```python
from build123d import *

# Parameters (mm, degrees)
SKETCH2_W           = 59.055
SKETCH2_H           = 25.4
BOSS_EXTRUDE1_DEPTH = 2
BOSS_EXTRUDE2_START = 2
BOSS_EXTRUDE2_DEPTH = 9.525
SKETCH3_W           = 38.1
SKETCH3_H           = 25.4
BOSS_EXTRUDE3_DEPTH = 2
BOSS_EXTRUDE4_START = 2
SKETCH4_W           = 3.175
SKETCH4_H           = 25.4
BOSS_EXTRUDE4_DEPTH = 6.35
SKETCH5_R           = 1.5875
CUT_EXTRUDE1_DEPTH  = 3.175
SKETCH6_W           = 35.56
SKETCH6_H           = 71.12
SKETCH6_R           = 1.5875
BOSS_EXTRUDE5_DEPTH = 2
FILLET1_R           = 2.54
SKETCH10_R          = 13.129221829
CUT_EXTRUDE2_DEPTH  = 2


with BuildPart() as part:
    # Sketch2 → Boss-Extrude1 (new body)
    with BuildSketch(Plane(origin=(0, 0, 0), x_dir=(1, 0, 0), z_dir=(0, 1, 0))):
        with Locations((26.9875, 154.94)):
            Rectangle(SKETCH2_W, SKETCH2_H)
    extrude(amount=BOSS_EXTRUDE1_DEPTH)

    # Sketch1 → Boss-Extrude2 (add)
    with BuildSketch(Plane(origin=(0, 0, 0), x_dir=(1, 0, 0), z_dir=(0, 1, 0)).offset(BOSS_EXTRUDE2_START)):
        Polygon((-2.54, 167.64), (-2.54, 158.115), (0, 158.115), (0, 165.1), (53.975, 165.1), (53.975, 158.115), (56.515, 158.115), (56.515, 167.64), align=None)
    extrude(amount=BOSS_EXTRUDE2_DEPTH)

    # Sketch3 → Boss-Extrude3 (add)
    with BuildSketch(Plane(origin=(0, 0, 0), x_dir=(1, 0, 0), z_dir=(0, 1, 0))):
        with Locations((75.565, 154.94)):
            Rectangle(SKETCH3_W, SKETCH3_H)
    extrude(amount=BOSS_EXTRUDE3_DEPTH)

    # Sketch4 → Boss-Extrude4 (add)
    with BuildSketch(Plane(origin=(0, 0, 0), x_dir=(1, 0, 0), z_dir=(0, 1, 0)).offset(BOSS_EXTRUDE4_START)):
        with Locations((93.0275, 154.94)):
            Rectangle(SKETCH4_W, SKETCH4_H)
    extrude(amount=BOSS_EXTRUDE4_DEPTH)

    # Sketch5 → Cut-Extrude1 (cut)
    with BuildSketch(Plane(origin=(94.615, 0, 0), x_dir=(0, 0, -1), z_dir=(1, 0, 0))):
        with Locations((145.94, 4.895971622)):
            Circle(SKETCH5_R)
        with Locations(Location((163.94, 4.895971622, 0), (0, 0, 180))):
            Circle(SKETCH5_R)
    extrude(amount=-CUT_EXTRUDE1_DEPTH, mode=Mode.SUBTRACT)

    # Mirror1: part across plane


with BuildPart() as part_1:
    add(part.part)
    add(part.part.mirror(Plane(origin=(26.9875, 0, 0), x_dir=(0, 0, 1), z_dir=(1, 0, 0))))

    # Sketch6 → Boss-Extrude5 (add)
    with BuildSketch(Plane(origin=(0, 0, 0), x_dir=(1, 0, 0), z_dir=(0, 1, 0))):
        with Locations((26.9875, 203.2)):
            Rectangle(SKETCH6_W, SKETCH6_H)
        with Locations(Location((11.09051688, 236.783908574, 0), (0, 0, 270))):
            Circle(SKETCH6_R, mode=Mode.SUBTRACT)
        with Locations(Location((11.09051688, 205.176091426, 0), (0, 0, 90))):
            Circle(SKETCH6_R, mode=Mode.SUBTRACT)
        with Locations(Location((42.88448312, 205.176091426, 0), (0, 0, 270))):
            Circle(SKETCH6_R, mode=Mode.SUBTRACT)
        with Locations(Location((42.88448312, 236.783908574, 0), (0, 0, 90))):
            Circle(SKETCH6_R, mode=Mode.SUBTRACT)
    extrude(amount=BOSS_EXTRUDE5_DEPTH)

    # Fillet1
    fillet1_edges = [part_1.edges().sort_by_distance(p)[0] for p in [
        (26.9875, 2, -167.64),
    ]]
    fillet(fillet1_edges, radius=FILLET1_R)

    # Sketch10 → Cut-Extrude2 (cut)
    with BuildSketch(Plane(origin=(0, 2, 0), x_dir=(1, 0, 0), z_dir=(0, 1, 0))):
        with Locations(Location((26.9875, 224.917, 0), (0, 0, 270))):
            Circle(SKETCH10_R)
    extrude(amount=-CUT_EXTRUDE2_DEPTH, mode=Mode.SUBTRACT)


solid = part_1.part
```
Could you check a few things on this model? Use its own coordinates, in mm. A direction names the side the tool comes from. Round coordinates to 2 decimals unless told otherwise and drop trailing zeros. Write each loop counter-clockwise with the first axis right and the second up, starting at its lowest first coordinate (ties: lowest second). Pieces come first, ordered by that corner, then holes. Notation, with made-up numbers: M -9.75,5 L 7.25,5 A32 cw 7.25,41 Z; hole C 17.25,77 d8. An arc over 180 degrees is marked long. Answer in a Markdown table with one row per item. Add a question column.
Q1. Imagine slicing it at C-C (z = -188.5). Please give me the cut outline in (x, y), then the cut area to 3 significant figures.
Q2. Will these pins go through, and if not, where does the flat tip stop? pin 1 Ø1 at (x, z) = (-38.5, -151.5) entering from +Y; pin 2 Ø3.5 at (y, z) = (4.9, -163.94) entering from -X; pin 3 Ø3 at (x, y) = (36.5, 8) entering from +Z; pin 4 Ø3 at (y, z) = (4.9, -163.94) entering from -X.
Q3. Imagine slicing it at A-A (z = -145.94). Please give me the cut outline in (x, y) (3 decimals), then the cut area to 3 significant figures.
Q4. If we mould it in two halves opening along X, with no side actions, what happens to faces 4 (the cylindrical face through (11.57, 0.99, -235.27)), 5 (the flat face through (44.768, 1, -203)), 6 (the cylindrical face through (93.05, 4.966, -144.354)), 7 (the flat face through (56.515, 7, -163))? For each: +X half, -X half, draft (parallel to the pull), parting line (faces both ways), or undercut.
Q5. Imagine slicing it at B-B (z = -232). Please give me the cut outline in (x, y).
Q6. Imagine slicing it at D-D (x = -21). Please give me the cut outline in (y, z).
Q7. If I drill on line 1 (X direction, y = 7.75, z = -163) (3 decimals); line 2 (Y direction, x = 38, z = -207.5); line 3 (Z direction, x = 6, y = 5.75), over which ranges is the centre line in solid material (lowest first)? Write a range as from..to.
Q8. On a 3-axis mill with a long thin cutter (end or side, diameter ignored), from which of +Z, -Z, +X, -X, +Y, -Y can I reach the whole of each face in a straight line? I mean faces 1 (the flat face through (0, 7, -162)), 2 (the flat face through (-2.54, 7, -163)), 3 (the cylindrical face through (-39.07, 5.86, -165.2)). Say none if no direction works.
Values:
| question | item | result |
|---|---|---|
| 1 | outline | M 9.21,0 L 44.77,0 L 44.77,2 L 9.21,2 Z |
| 1 | area | 71.1 mm^2 |
| 2 | pin 1 | y = 8.35 |
| 2 | pin 2 | x = -40.64 |
| 2 | pin 3 | z = -165.1 |
| 2 | pin 4 | x = -2.54 |
| 3 | outline | M -40.64,0 L 94.615,0 L 94.615,3.308 L 91.44,3.308 L 91.44,2 L -37.465,2 L -37.465,3.308 L -40.64,3.308 Z; M -40.64,6.483 L -37.465,6.483 L -37.465,8.35 L -40.64,8.35 Z; M 91.44,6.483 L 94.615,6.483 L 94.615,8.35 L 91.44,8.35 Z |
| 3 | area | 291 mm^2 |
| 4 | face 4 | undercut |
| 4 | face 5 | +X half |
| 4 | face 6 | draft |
| 4 | face 7 | undercut |
| 5 | outline | M 9.21,0 L 15.93,0 L 15.93,2 L 9.21,2 Z; M 38.04,0 L 44.77,0 L 44.77,2 L 38.04,2 Z |
| 6 | outline | M 0,-167.64 L 2,-167.64 L 2,-142.24 L 0,-142.24 Z |
| 7 | line 1 | -40.64..-37.465, -2.54..0, 53.975..56.515, 91.44..94.615 |
| 7 | line 2 | 0..2 |
| 7 | line 3 | -167.64..-165.1 |
| 8 | face 1 | +Z, +Y |
| 8 | face 2 | +Z, -Z, +Y |
| 8 | face 3 | -X |
